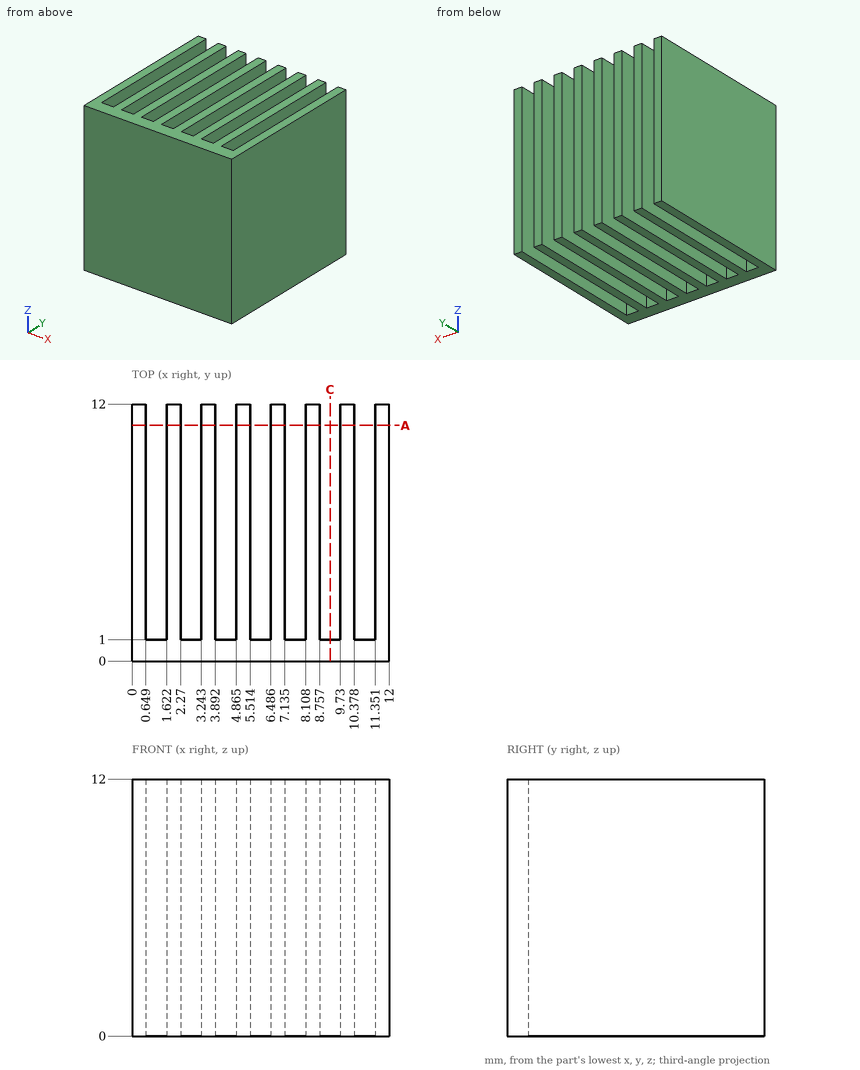
Can you work these out from the drawing? Everything is in mm from the part's minimum corner. Coordinates: 2 decimals unless noted, no trailing zeros. Loops run counter-clockwise (first coordinate to the right, second up) from the corner with the lowest first, then second, coordinate; pieces in that order, holes last.
1) For pin 1 (0.5 mm diameter, centred on x = 4.5, z = 5, fed in from +Y), with a flat end and sliding along its axis, tell me the tip position at first contact or that it passes through.
2) I need wall thicknesses on probe 1 along Y at (x, z) = (4, 10). Which ranges of the line are inside material? Lowest first, please.
3) Imagine slicing it at A-A on y = 11. State how many separate pieces and enclosed holes the cut face has.
4) Imagine slicing it at C-C on x = 9.25. List the corners of the cut face in (y, z) for me.
Completed:
1. pin 1: stops at y = 1
2. probe 1: y = 0 to 1
3. separate pieces: 8
3. enclosed holes: 0
4. outline: (0, 0) - (1, 0) - (1, 12) - (0, 12) - close
